Answer from the drawing. Dimensions are ordinates in mm from the lowest x, y and z of the part. A direction names the side the tool comes from. Coordinates: 2 decimals unless noted, no trailing zeros. Write each loop counter-clockwise with the first axis right and the second up, starting at its lowest first coordinate (ties: lowest second). Pieces come first, ordered by that corner, then holes.
(1) Given pin 1 (2.5 mm diameter, centred on y = 29, z = 73, fed in from -X); pin 2 (12.5 mm diameter, centred on x = 122, y = 25, fed in from -Z) (3 decimals); pin 3 (12.5 mm diameter, centred on x = 103, y = 27, fed in from -Z), each flat-ended and moving along its own axis, determine where each tip first touches the part or whether it passes through.
(2) Find the intervals of material crossed by probe 1 along Z at (x, y) = (105, 32); probe 2 along Z at (x, y) = (126, 34) (3 decimals); probe 3 along X at (y, z) = (35, 23), in increasing order.
(3) The mould has two halves that part along X. Classify the marked faces 1, 2 and 3: +X half, -X half, draft (parallel to the pull), parting line (faces both ways), or undercut.
(4) Which of the six approach directions +Z, -Z, +X, -X, +Y, -Y give full straight-line access (tool end or side, diameter ignored) to the marked faces 4, 5 and 6?
(5) Section C-C on z = 8.5 is taken. Write down the section's boundary in (x, y), then the cut area to 3 significant figures.
(6) Section B-B on x = 15.5 is taken. Write down the section's boundary in (y, z).
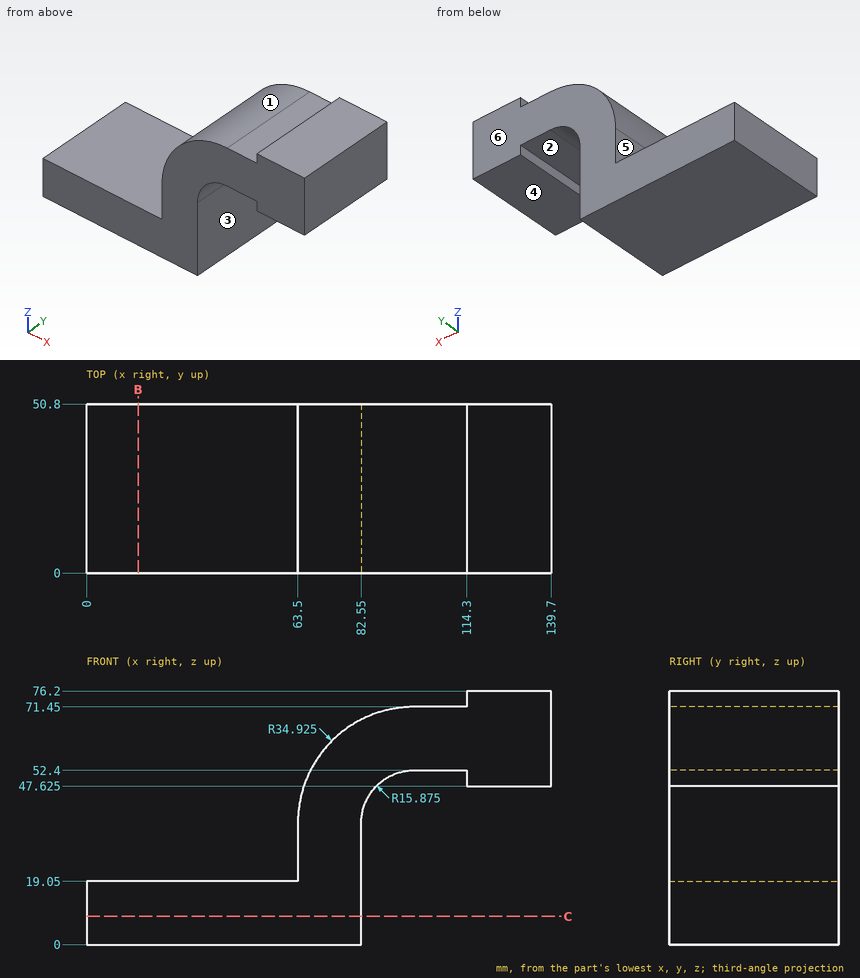
Response:
1. pin 1: stops at x = 114.3
1. pin 2: stops at z = 47.625
1. pin 3: stops at z = 52.31
2. probe 1: z = 52.4 to 71.45
2. probe 2: z = 47.625 to 76.2
2. probe 3: x = 63.5 to 82.55
3. face 1: -X half
3. face 2: undercut
3. face 3: +X half
4. face 4: -Z, +X, +Y, -Y
4. face 5: +Z, -X, +Y, -Y
4. face 6: +Z, -Z, +X, -X, +Y
5. outline: (0, 0) - (82.55, 0) - (82.55, 50.8) - (0, 50.8) - close
5. area: 4,190 mm2
6. outline: (0, 0) - (50.8, 0) - (50.8, 19.05) - (0, 19.05) - close
